from build123d import *

# Parameters (mm, degrees)
BOSS_EXTRUDE3_DEPTH     = 12.5
SKETCH6_R               = 2.35
CUT_EXTRUDE1_DEPTH      = 38.225
CUT_EXTRUDE1_DEPTH_BACK = 34.45
CHAMFER1_SIZE           = 0.5


with BuildPart() as part:
    # Sketch5 → Boss-Extrude3 (new body, symmetric)
    with BuildSketch(Plane.XY):
        with BuildLine():
            Line((33.45, 0.7), (37.225, 4.475))
            Line((37.225, 4.475), (37.225, 15.7))
            Line((37.225, 15.7), (32.225, 15.7))
            Line((32.225, 15.7), (32.225, 7.7))
            ThreePointArc((32.225, 7.7), (31.932106781, 6.992893219), (31.225, 6.7))
            Line((31.225, 6.7), (-10.775, 6.7))
            ThreePointArc((-10.775, 6.7), (-11.482106781, 6.992893219), (-11.775, 7.7))
            Line((-11.775, 7.7), (-11.775, 15.7))
            Line((-11.775, 15.7), (-16.775, 15.7))
            Line((-16.775, 15.7), (-16.775, 7.7))
            ThreePointArc((-16.775, 7.7), (-17.067893219, 6.992893219), (-17.775, 6.7))
            Line((-17.775, 6.7), (-32.45, 6.7))
            ThreePointArc((-32.45, 6.7), (-33.157106781, 6.407106781), (-33.45, 5.7))
            Line((-33.45, 5.7), (-33.45, -9.3))
            Line((-33.45, -9.3), (-28.45, -9.3))
            Line((-28.45, -9.3), (-28.45, 0.7))
            Line((-28.45, 0.7), (28.45, 0.7))
            Line((28.45, 0.7), (28.45, -9.3))
            Line((28.45, -9.3), (33.45, -9.3))
            Line((33.45, -9.3), (33.45, 0.7))
        make_face()
    extrude(amount=BOSS_EXTRUDE3_DEPTH, both=True)

    # Sketch6 → Cut-Extrude1 (cut, two sides)
    with BuildSketch(Plane(origin=(0, 0, 0), x_dir=(0, 0, -1), z_dir=(1, 0, 0))) as cut_extrude1_sk:
        with Locations((-4.25, 11.05)):
            Circle(SKETCH6_R)
        with Locations((4.25, 11.05)):
            Circle(SKETCH6_R)
        with Locations((4.25, -5.3)):
            Circle(SKETCH6_R)
        with Locations((-4.25, -5.3)):
            Circle(SKETCH6_R)
    extrude(amount=CUT_EXTRUDE1_DEPTH, mode=Mode.SUBTRACT)
    extrude(cut_extrude1_sk.sketch, amount=-CUT_EXTRUDE1_DEPTH_BACK, mode=Mode.SUBTRACT)

    # Chamfer1
    chamfer1_edges = [part.edges().sort_by_distance(p)[0] for p in [
        (-11.775, 15.7, 0),
        (32.225, 15.7, 0),
        (28.45, -9.3, 0),
        (-28.45, -9.3, 0),
    ]]
    chamfer(chamfer1_edges, length=CHAMFER1_SIZE)


solid = part.part
Geometry: final body of the model. Coordinates: model frame, mm. A direction names the side the tool comes from. Coordinates: 2 decimals unless noted, no trailing zeros. Loops run counter-clockwise (first coordinate to the right, second up) from the corner with the lowest first, then second, coordinate; pieces in that order, holes last. Notation, with made-up numbers: (48.25, -11.75) - (101.25, -11.75) arc R22 cw to (101.25, 1.25) - close; hole circle Ø10 at (7.25, 48.5). An arc over 180 degrees is marked (long way). One line per question, with ' | ' between items. Start each with the question number.
(1) Draft query along Y for faces 5 (the flat face through (11, 6.7, 0)), 6 (the cylindrical face through (-30.915, -3.318, -5.513)), 7 (the flat face through (1, 3, 12.5)). Return one class per face: +Y half, -Y half, draft (parallel to the pull), parting line (faces both ways), or undercut.
(2) Cut plane C-C on x = -3. Output: boundary loops of the cut face in (y, z).
(3) Cut plane A-A on y = 11.05. Output: boundary loops of the cut face in (x, z) (3 decimals).
(4) Ray query, L1, parallel to Z at x = 33.45, y = 11.05; L2, parallel to X at y = -7, z = -10; L3, parallel to X at y = 13.25, z = 7 (3 decimals). Return the intervals inside material, ascending. Write a range as from..to.
(5) First-contact query: pin 1 (4 mm diameter, centred on x = 8, z = 0, fed in from +Y); pin 2 (1.5 mm diameter, centred on x = 4.5, z = 9.5, fed in from -Y); pin 3 (7.5 mm diameter, centred on y = 11.05, z = 4.25, fed in from -X). Flat tips, straight axial feed; report the tip coordinate or a pass-through.
(6) Reachability of faces 1 (the flat face through (-25, 6.7, 0)), 2 (the flat face through (-11.775, 11, 0)), 3 (the flat face through (28.45, -4, 0)), 4 (the flat face through (33.45, -4, 0)) from +Z, -Z, +X, -X, +Y, -Y: full face, straight path, thin tool, end or side. Return the list, or none.
(7) Cut plane B-B on z = -4.25. Count the separate pieces of the cut face and the enclosed holes in it, and give its area (3 significant figures).
Here are the results:
1) face 5: +Y half | face 6: undercut | face 7: draft
2) outline: (0.7, -12.5) - (6.7, -12.5) - (6.7, 12.5) - (0.7, 12.5) - close
3) outline: (-16.775, -12.5) - (-11.775, -12.5) - (-11.775, -6.6) - (-16.775, -6.6) - close; (-16.775, -1.9) - (-11.775, -1.9) - (-11.775, 1.9) - (-16.775, 1.9) - close; (-16.775, 6.6) - (-11.775, 6.6) - (-11.775, 12.5) - (-16.775, 12.5) - close; (32.225, -12.5) - (37.225, -12.5) - (37.225, -6.6) - (32.225, -6.6) - close; (32.225, -1.9) - (37.225, -1.9) - (37.225, 1.9) - (32.225, 1.9) - close; (32.225, 6.6) - (37.225, 6.6) - (37.225, 12.5) - (32.225, 12.5) - close
4) L1: -12.5..-6.6, -1.9..1.9, 6.6..12.5 | L2: -33.45..-28.45, 28.45..33.45 | L3: -16.775..-11.775, 32.225..37.225
5) pin 1: y = 6.7 | pin 2: y = 0.7 | pin 3: x = -16.86
6) face 1: +Z, -Z, -X, +Y | face 2: +Z, -Z, +Y | face 3: +Z, -Z, -Y | face 4: +Z, -Z, +X, -Y
7) separate pieces: 5 | enclosed holes: 0 | area: 513 mm²
